Autodesk Inventor part; units mm, degrees
ref_plane "YZ Plane" through (0, 0, 0) normal (1, 0, 0) x (0, 1, 0)
ref_plane "XZ Plane" through (0, 0, 0) normal (0, 1, 0) x (-1, 0, 0)
ref_plane "XY Plane" through (0, 0, 0) normal (0, 0, 1) x (1, 0, 0)
sketch "Esquisse1" plane through (0, 0, 0) normal (0, 0, 1) x (1, 0, 0)
  circle A0 centre (0, 0) radius 3.75
  dimension "d0" = 7.5
extrude "Extrusion1" add sketch "Esquisse1" along normal blind 5
sketch "Esquisse3" plane through (0, 0, 5) normal (0, 0, 1) x (1, 0, 0)
  circle A0 centre (0, 0) radius 5
  dimension "d12" = 10
extrude "Extrusion2" add sketch "Esquisse3" along normal blind 5
sketch "Esquisse4" plane through (0, 0, 10) normal (0, 0, 1) x (1, 0, 0)
  circle A0 centre (0, 0) radius 3.75
  circle A1 centre (0, 0) radius 5
  circle A2 centre (0, 0) radius 3.75
  line L0 (0, 3.75) -> (-0.9296, 4.9771)
  line L1 (-0.9296, 4.9771) -> (-1, 5.07)
  line L2 (-1, 5.07) -> (1, 5.07)
  line L3 (1, 5.07) -> (0, 3.75)
  dimension "d15" = 7.5
  dimension "d16" = 2
  dimension "d17" = 1.32
  dimension "d18" = 1
extrude "Extrusion3" cut sketch "Esquisse4" against normal blind 5 contours L0 A1 L3 | L0 L1 L2 L3 A1 picked at (0.3946, 4.554)
pattern_circular "Réseau circulaire1" count 18 over 360 about axis through (0, 0, 5) along (0, 0, 1) of "Extrusion3"
sketch "Esquisse5" plane through (0, 0, 10) normal (0, 0, 1) x (1, 0, 0)
  circle A0 centre (0, 0) radius 1.2
  dimension "d24" = 2.4
extrude "Extrusion4" cut sketch "Esquisse5" against normal through all
sketch "Esquisse6" plane through (0, 0, 0) normal (1, 0, 0) x (0, 1, 0)
  circle A0 centre (0, 3) radius 1.5
  line L0 (-3.75, 0) -> (3.75, 0)
  point P0 (0, 0)
  dimension "d27" = 3
  dimension "d28" = 3
extrude "Extrusion5" cut sketch "Esquisse6" against normal blind 5
properties part number "Pignon" material "Laiton, jaune doux, soudé"
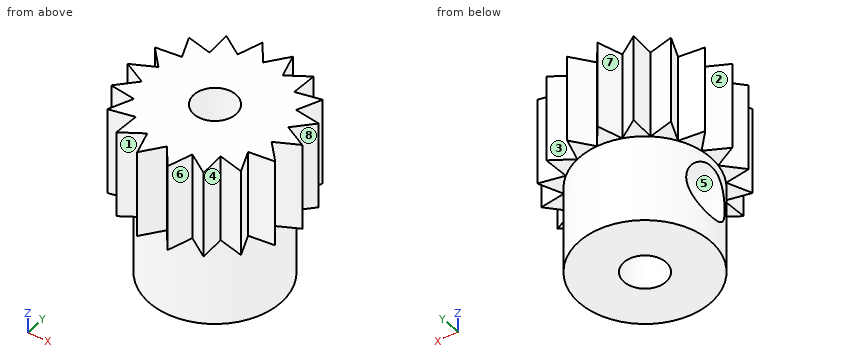
Work out the finished part from the listing and answer in its coordinate system (mm). Face numbers are marked on the shaded views. A direction names the side the tool comes from. Coordinates: 2 decimals unless noted, no trailing zeros. Write each loop counter-clockwise with the first axis right and the second up, starting at its lowest first coordinate (ties: lowest second). Pieces come first, ordered by that corner, then holes.
Q1. A cutting plane is placed at B-B, the plane x = 1.5. Give the vertices of the cut face in (y, z), then the cut area to 3 significant figures.
Q2. A cutting plane is placed at A-A, the plane z = 4.75. Give the vertices of the cut face in (x, y), then the cut area to 3 significant figures.
Q3. A cutting plane is placed at C-C, the plane z = 3. Give the vertices of the cut face in (x, y), then the cut area to 3 significant figures.
Q4. Determine the mould class of the marked faces 5, 6, 7 and 8 for opening direction Y: released by +Y, released by -Y, zero draft, split by the parting line, or undercut.
Q5. Which of the six approach directions +Z, -Z, +X, -X, +Y, -Y give full straight-line access (tool end or side, diameter ignored) to the marked faces 1, 2, 3 and 4?
Q6. Each of these flat-tipped pins is pushed along its axis until it touches: pin 1 Ø4 at (y, z) = (2, 4.5) entering from -X; pin 2 Ø1.3 at (x, y) = (-3.5, 1.5) entering from -Z; pin 3 Ø1.5 at (x, z) = (1.5, 3.5) entering from +Y; pin 4 Ø1 at (x, y) = (0.5, 4.5) entering from -Z. Where does it stop, or does it pass through?
Q7. Find the intervals of material crossed by line 1 (Y direction, x = 0, z = 4.75); line 2 (X direction, y = 0, z = 4); line 3 (Z direction, x = -3, y = -0.75), in increasing order.
Findings below:
1. outline: (-3.66, 5) - (-3.44, 5) - (-3.44, 0) - (3.44, 0) - (3.44, 5) - (3.66, 5) - (3.66, 10) - (-3.66, 10) - close
1. area: 71.0 mm2
2. outline: circle Ø7.5 at (0, 0); hole circle Ø2.4 at (0, 0)
2. area: 39.7 mm2
3. outline: (-3.44, -1.5) arc R3.75 ccw (long way) to (-3.44, 1.5) - (0, 1.5) - (0, 1.2) arc R1.2 cw to (0, -1.2) - (0, -1.5) - close
3. area: 31.0 mm2
4. face 5: undercut
4. face 6: released by -Y
4. face 7: released by +Y
4. face 8: undercut
5. face 1: +Z, -Z, -Y
5. face 2: +Z, -Z, -X
5. face 3: +Z, -Z, +Y
5. face 4: +Z, -Z
6. pin 1: stops at x = -4.84
6. pin 2: stops at z = 0
6. pin 3: stops at y = 3.67
6. pin 4: stops at z = 5
7. line 1: y = -3.75 to -1.2, 1.2 to 3.75
7. line 2: x = 1.2 to 3.75
7. line 3: z = 0 to 1.7, 4.3 to 10
